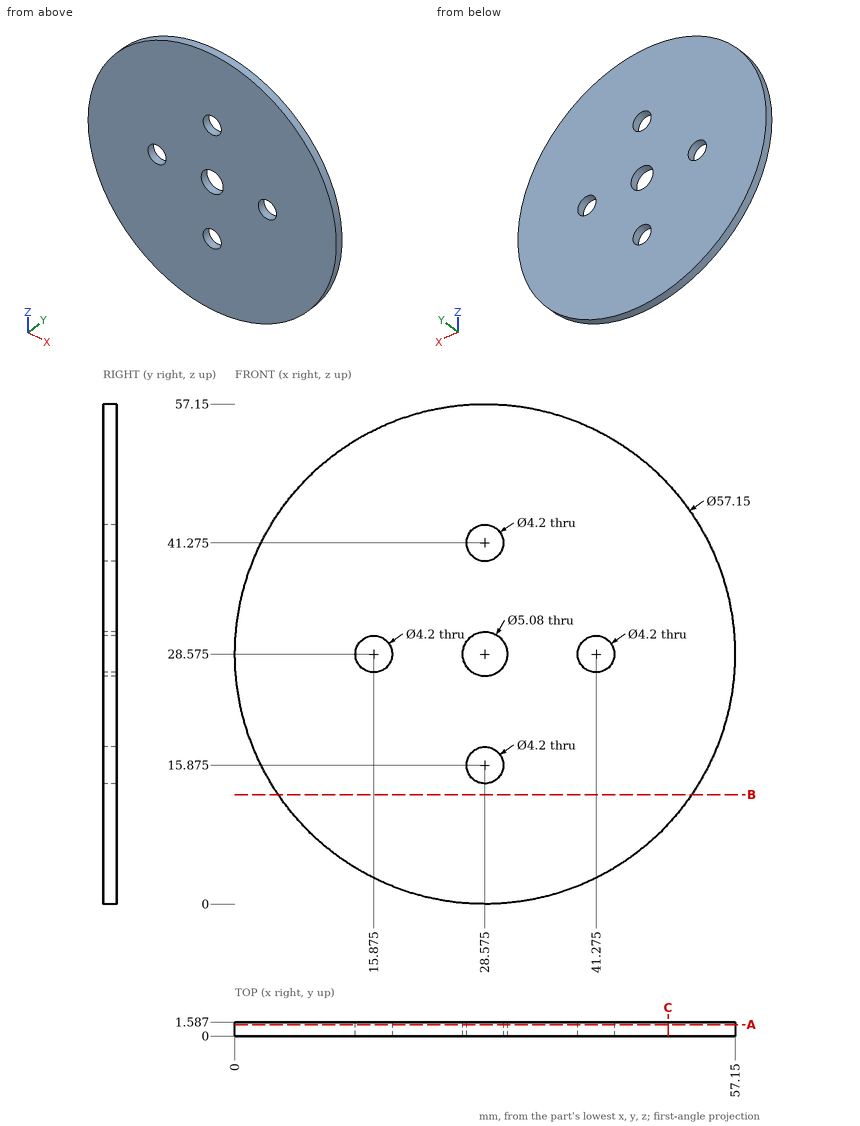
Could you check a few things on this drawing? It's one solid part, dimensions in mm from its lowest x, y, z. Give positions to 0.01 mm unless a question says otherwise; leave off trailing zeros. Order: outer loops, then holes, each group sorted by start corner. A loop starts at its lowest first (then second) coordinate and runs counter-clockwise, first axis right, second up. Notation, with made-up numbers: (17, -33) - (70, -33) arc R9 ccw to (70, -27) - close; hole circle Ø4 at (87.25, 37). An arc over 180 degrees is marked (long way). Return JSON: item names as keys, results as strings. Group by question number.
Q1. Suppose I cut it at B-B, the plane z = 12.5. Please give me the cut outline in (x, y).
Q2. Will this pin go through, and if not, where does the flat tip stop? pin 1 Ø2.5 at (x, z) = (28.575, 15.875) entering from -Y.
Q3. Please list where these lines run through material, in increasing order: line 1 along Z through (x, y) = (17, 0.75); line 2 along X through (y, z) = (0.8, 43) (1 decimal); line 3 along Z through (x, y) = (16.5, 1.2) (1 decimal). Write a range as [from, to].
Q4. Suppose I cut it at A-A, the plane y = 1.3. State how many separate pieces and enclosed holes the cut face has, and give its area (3 significant figures).
Q5. Suppose I cut it at C-C, the plane x = 49.5. Please give me the cut outline in (y, z) (1 decimal).
Resolved:
{
 "1": {"outline": "(4.95, 0) - (52.2, 0) - (52.2, 1.59) - (4.95, 1.59) - close"},
 "2": {"pin 1": "passes through"},
 "3": {"line 1": "z = [2.45, 26.8], [30.35, 54.7]", "line 2": "x = [3.9, 27.4], [29.8, 53.2]", "line 3": "z = [2.7, 26.6], [30.6, 54.5]"},
 "4": {"separate pieces": "1", "enclosed holes": "5", "area": "2,490 mm2"},
 "5": {"outline": "(0, 9.1) - (1.6, 9.1) - (1.6, 48) - (0, 48) - close"}
}
